Study the drawing (mm; zero at the part's minimum x, y, z) and answer. Give positions to 0.01 mm unless a question says otherwise; leave off trailing zeros. Order: outer loops, then holes, each group sorted by start corner. A loop starts at its lowest first (then second) coordinate and runs counter-clockwise, first axis right, second up. Notation, with made-up numbers: (-27.75, 20) - (3.25, 20) arc R29 cw to (3.25, 44) - close; hole circle Ø5 at (17.25, -7). An arc over 180 degrees is marked (long way). Return JSON: item names as keys, results as strings.
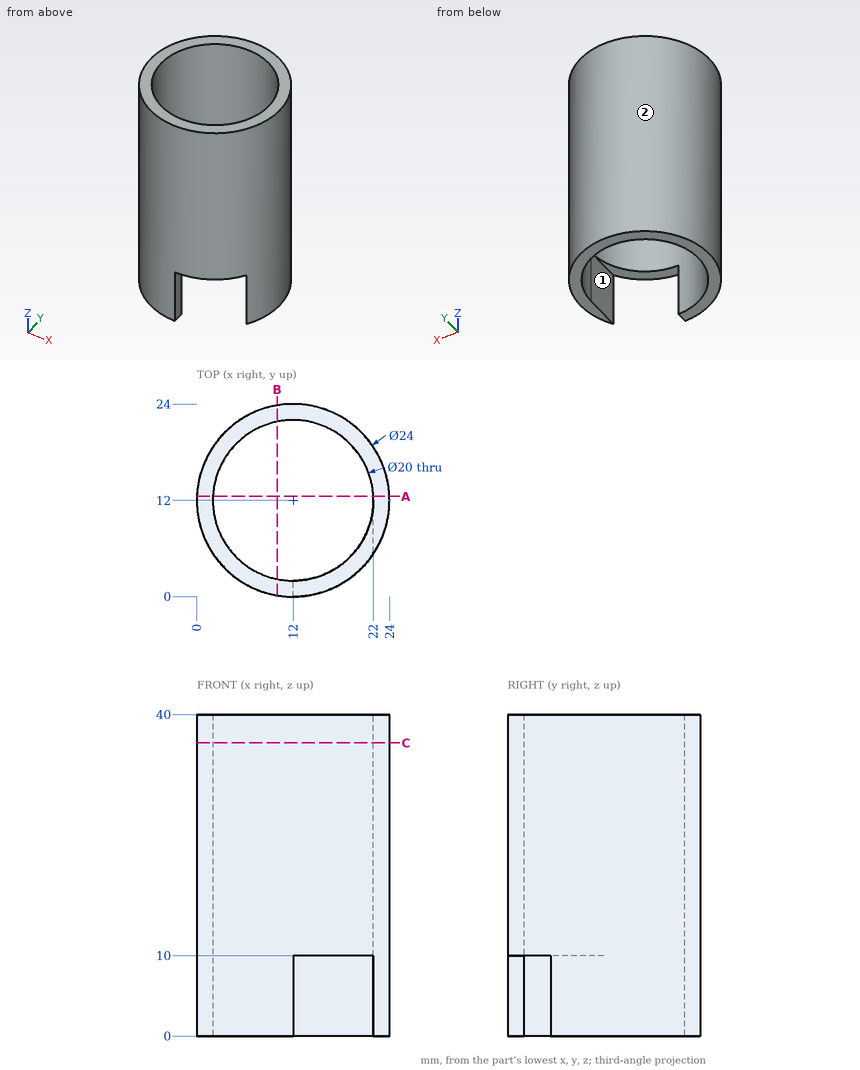
Q1. Given pin 1 (12 mm diameter, centred on x = 18, z = 26, fed in from +Y); pin 2 (5 mm diameter, centred on x = 19.5, z = 13, fed in from -Y); pin 3 (0.6 mm diameter, centred on y = 1, z = 3, fed in from +X); pin 4 (5.5 mm diameter, centred on y = 8, z = 3.5, fed in from -X), each flat-ended and moving along its own axis, determine where each tip first touches the part or whether it passes through.
Values:
{"pin 1": "stops at y = 24", "pin 2": "stops at y = 1.09", "pin 3": "stops at x = 12", "pin 4": "stops at x = 0.07"}
Q2. Consider L1, parallel to Y at x = 12, z = 29; L2, parallel to Y at x = 9, z = 9.5. Determine where each line is inside the solid, lowest interval first.
Values:
{"L1": "y = 0 to 2, 22 to 24", "L2": "y = 0.38 to 2.46, 21.54 to 23.62"}
Q3. Determine the mould class of the marked faces 1 and 2 for opening direction X: released by +X, released by -X, zero draft, split by the parting line, or undercut.
Values:
{"face 1": "undercut", "face 2": "split by the parting line"}
Q4. A cutting plane is placed at C-C (z = 36.5). Write down the section's boundary in (x, y), and give its area (3 significant figures).
Values:
{"outline": "circle Ø24 at (12, 12); hole circle Ø20 at (12, 12)", "area": "138 mm²"}
Q5. A cutting plane is placed at B-B (x = 10). Write down the section's boundary in (y, z), and give its area (3 significant figures).
Values:
{"outline": "(0.17, 0) - (2.2, 0) - (2.2, 40) - (0.17, 40) - close; (21.8, 0) - (23.83, 0) - (23.83, 40) - (21.8, 40) - close", "area": "163 mm²"}
Q6. A cutting plane is placed at A-A (y = 12.5). Write down the section's boundary in (x, z), and give its area (3 significant figures).
Values:
{"outline": "(0.01, 0) - (2.01, 0) - (2.01, 40) - (0.01, 40) - close; (21.99, 0) - (23.99, 0) - (23.99, 40) - (21.99, 40) - close", "area": "160 mm²"}
